```python
from build123d import *

# Parameters (mm, degrees)
SKETCH1_W           = 1000
SKETCH1_H           = 580
BOSS_EXTRUDE1_DEPTH = 10
SKETCH2_W           = 440
SKETCH2_H           = 480
CUT_EXTRUDE3_DEPTH  = 795.596872652
SHELL2_START        = -593.858216583
SHELL2_OUTLINE_W    = 48
SHELL2_OUTLINE_H    = 8
SHELL2_DEPTH        = 998
SHELL2_START_2      = -153.858216583
SHELL2_2_OUTLINE_W  = 482
SHELL2_2_OUTLINE_H  = 8
SHELL2_2_DEPTH      = 118
BOSS_EXTRUDE2_DEPTH = 3
BOSS_EXTRUDE4_DEPTH = 3
SKETCH11_R          = 5
CUT_EXTRUDE6_DEPTH  = 799.473143596
SKETCH13_R          = 5
CUT_EXTRUDE7_DEPTH  = 799.473143596
SKETCH14_W          = 20
SKETCH14_H          = 60
BOSS_EXTRUDE5_DEPTH = 10
SKETCH15_W          = 20
SKETCH15_H          = 60
BOSS_EXTRUDE6_DEPTH = 10


# Read off the part's stored shape, not the designer's step: Shell2
with BuildPart() as part:
    # Sketch1 → Boss-Extrude1 (new body)
    with BuildSketch(Plane.XY):
        with Locations((-94.858216583, -236.714241493)):
            Rectangle(SKETCH1_W, SKETCH1_H)
    extrude(amount=BOSS_EXTRUDE1_DEPTH)

    # Sketch2 → Cut-Extrude3 (cut, through all)
    with BuildSketch(Plane.XY.offset(10)):
        with Locations((185.141783417, -236.714241493)):
            Rectangle(SKETCH2_W, SKETCH2_H)
        with Locations((-374.858216583, -236.714241493)):
            Rectangle(SKETCH2_W, SKETCH2_H)
    extrude(amount=-CUT_EXTRUDE3_DEPTH, mode=Mode.SUBTRACT)

    # Shell2 outline → Shell2 (cut)
    with BuildSketch(Plane.YZ.offset(SHELL2_START)):
        with Locations((-501.714241493, 5)):
            Rectangle(SHELL2_OUTLINE_W, SHELL2_OUTLINE_H)
        with Locations((28.285758507, 5)):
            Rectangle(SHELL2_OUTLINE_W, SHELL2_OUTLINE_H)
    extrude(amount=SHELL2_DEPTH, mode=Mode.SUBTRACT)

    # Shell2 2 outline → Shell2 2 (cut)
    with BuildSketch(Plane.YZ.offset(SHELL2_START_2)):
        with Locations((-236.714241493, 5)):
            Rectangle(SHELL2_2_OUTLINE_W, SHELL2_2_OUTLINE_H)
    extrude(amount=SHELL2_2_DEPTH, mode=Mode.SUBTRACT)

    # Sketch5 → Boss-Extrude2 (add)
    with BuildSketch(Plane(origin=(0, -476.714241493, 0), x_dir=(1, 0, 0), z_dir=(0, 1, 0))):
        Polygon((405.141783417, 0), (431.885950294, -42.246296146), (414.987431836, -52.943962897), (366.847931456, 23.099370165), (383.746449915, 33.797036917), align=None)
    extrude(amount=-BOSS_EXTRUDE2_DEPTH)

    # Sketch10 → Boss-Extrude4 (add)
    with BuildSketch(Plane.XZ.offset(-3.285758507)):
        Polygon((405.141783417, 0), (431.885972414, 42.246282142), (414.987459557, 52.943957741), (366.847919362, -23.099350115), (383.746432219, -33.797025714), align=None)
    extrude(amount=-BOSS_EXTRUDE4_DEPTH)

    # Sketch11 → Cut-Extrude6 (cut, through all)
    with BuildSketch(Plane.XZ.offset(-3.285758507)):
        with Locations(Location((415.58302294, 35.189085408, 0), (0, 0, 270))):
            Circle(SKETCH11_R)
        with Locations(Location((384.0775579, -14.578315099, 0), (0, 0, 270))):
            Circle(SKETCH11_R)
    extrude(amount=-CUT_EXTRUDE6_DEPTH, mode=Mode.SUBTRACT)

    # Sketch13 → Cut-Extrude7 (cut, through all)
    with BuildSketch(Plane(origin=(0, -476.714241493, 0), x_dir=(1, 0, 0), z_dir=(0, 1, 0))):
        with Locations(Location((413.151340982, -31.347925129, 0), (0, 0, 180))):
            Circle(SKETCH13_R)
        with Locations(Location((384.72142187, 13.561261525, 0), (0, 0, 180))):
            Circle(SKETCH13_R)
    extrude(amount=-CUT_EXTRUDE7_DEPTH, mode=Mode.SUBTRACT)

    # Sketch14 → Boss-Extrude5 (add)
    with BuildSketch(Plane.ZY.offset(594.858216583)):
        with Locations((5, 28.285758507)):
            Rectangle(SKETCH14_W, SKETCH14_H)
    extrude(amount=-BOSS_EXTRUDE5_DEPTH)

    # Sketch15 → Boss-Extrude6 (add)
    with BuildSketch(Plane.ZY.offset(594.858216583)):
        with Locations((5, -501.714241493)):
            Rectangle(SKETCH15_W, SKETCH15_H)
    extrude(amount=-BOSS_EXTRUDE6_DEPTH)


solid = part.part
```
Geometry: final body of the model. Coordinates: model frame, mm. A direction names the side the tool comes from. Give positions to 0.01 mm unless a question says otherwise; leave off trailing zeros. Write each loop counter-clockwise with the first axis right and the second up, starting at its lowest first coordinate (ties: lowest second). Pieces come first, ordered by that corner, then holes.
1. Section query B-B, the plane y = -299.5. Return loops of the section in (x, z).
2. Reachability of faces 1 (the flat face through (-93, -238, 1)), 2 (the flat face through (232, 3.286, 7)), 3 (the flat face through (-594.858, 29, 5)), 4 (the flat face through (386, 6.286, -9)) from +Z, -Z, +X, -X, +Y, -Y: full face, straight path, thin tool, end or side. Return the list, or none.
3. Draft query along Y for faces 5 (the flat face through (391, -479.714, -13)), 6 (the flat face through (-92, -235, 10)), 7 (the flat face through (251, -476.714, 6)). Return one class per face: released by +Y, released by -Y, zero draft, split by the parting line, or undercut.
4. Pin query (flat end, axial travel): P1, Ø2.5, axis at y = 33, z = 5, coming from the +X side; P2, Ø5, axis at x = -315, z = 2.5, coming from the -Y side; P3, Ø6.5, axis at y = -213, z = 5.5, coming from the -X side. Return the tip coordinate at first contact, or that it passes through.
5. Section query C-C, the plane x = -118. Return loops of the section in (y, z), then the cut area to 3 significant figures.
6. Section query A-A, the plane x = -519.5. Return loops of the section in (y, z).
7. Line query: probe 1 along Y at (x, z) = (-287, 4.5); probe 2 along X at (y, z) = (-381, 3); probe 3 along Y at (x, z) = (380.5, -28.5). Output: solid intervals per line, ascending.
Computed:
1. outline: (-154.86, 0) - (-34.86, 0) - (-34.86, 10) - (-154.86, 10) - close; hole (-153.86, 1) - (-35.86, 1) - (-35.86, 9) - (-153.86, 9) - close
2. face 1: none
2. face 2: +Z, -Z, +X
2. face 3: +Z, -Z, -X, +Y, -Y
2. face 4: -Z, +X, +Y
3. face 5: released by -Y
3. face 6: zero draft
3. face 7: undercut
4. P1: stops at x = 405.14
4. P2: stops at y = -526.71
4. P3: stops at x = -154.86
5. outline: (-526.71, 0) - (53.29, 0) - (53.29, 10) - (-526.71, 10) - close; hole (-525.71, 1) - (52.29, 1) - (52.29, 9) - (-525.71, 9) - close
5. area: 1,180 mm2
6. outline: (-526.71, 0) - (-476.71, 0) - (-476.71, 10) - (-526.71, 10) - close; (3.29, 0) - (53.29, 0) - (53.29, 10) - (3.29, 10) - close; hole (-525.71, 1) - (-477.71, 1) - (-477.71, 9) - (-525.71, 9) - close; hole (4.29, 1) - (52.29, 1) - (52.29, 9) - (4.29, 9) - close
7. probe 1: y = -526.71 to -525.71, -477.71 to -476.71, 3.29 to 4.29, 52.29 to 53.29
7. probe 2: x = -154.86 to -153.86, -35.86 to -34.86
7. probe 3: y = -479.71 to -476.71, 3.29 to 6.29
